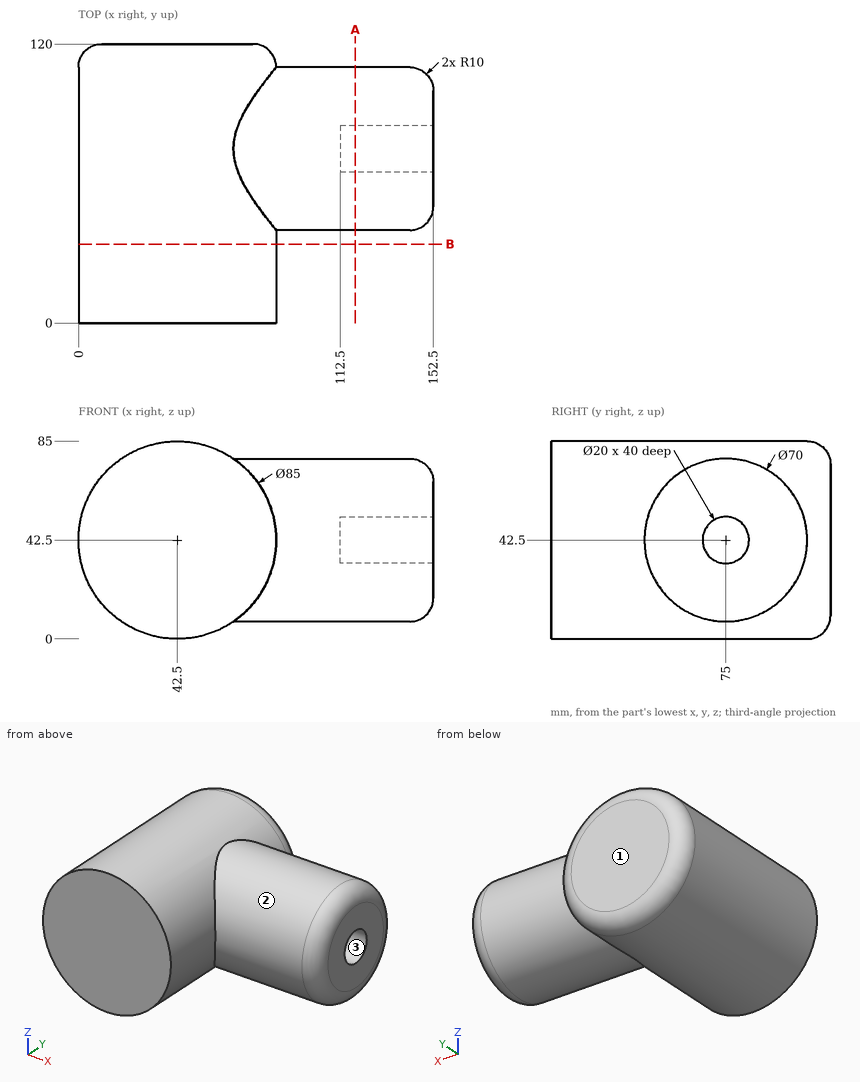
Study the drawing (mm; zero at the part's minimum x, y, z) and answer. Give positions to 0.01 mm unless a question says otherwise; leave off trailing zeros. Loops run counter-clockwise (first coordinate to the right, second up) from the corner with the lowest first, then second, coordinate; pieces in that order, holes last. Notation, with made-up numbers: M 54,21 L 72,21 A23 cw 72,41 Z; hole C 81,-28.5 d10. An arc over 180 degrees is marked long. One line per item, written item: value.
1. Section B-B on y = 34 is taken. Determine the outline of the cut face in (x, z), plus the area to 3 significant figures.
Found:
outline: C 42.5,42.5 d85
area: 5,670 mm^2
2. Find the intervals of material crossed by probe 1 along Y at (x, z) = (122, 42.5); probe 2 along Y at (x, z) = (101, 42); probe 3 along Z at (x, y) = (43, 92.5), in increasing order.
Found:
probe 1: 40 to 65, 85 to 110
probe 2: 40 to 110
probe 3: 0 to 85
3. Each of these flat-tipped pins is pushed along its axis until it touches: P1, Ø16, axis at y = 73, z = 43, coming from the +X side; P2, Ø4, axis at x = 18.5, y = 71.5, coming from the +Z side; P3, Ø1.5, axis at y = 29.5, z = 24.5, coming from the -X side; P4, Ø1.5, axis at x = 38.5, y = 49, coming from the -Z side. Where does it stop, or does it pass through?
Found:
P1: x = 152.5
P2: z = 78.86
P3: x = 3.66
P4: z = 0.12
4. Section A-A on x = 119 is taken. Determine the outline of the cut face in (y, z), plus the area to 3 significant figures.
Found:
outline: C 75,42.5 d70; hole C 75,42.5 d20
area: 3,530 mm^2
5. For a pull along Z with two mould halves and no side action, classify the marked faces 1, 2 and 3 as pulls with the +Z half, pulls with the -Z half, needs draft (parallel to the pull), parting line crosses it, or undercut.
Found:
face 1: needs draft
face 2: parting line crosses it
face 3: undercut
